Work out the finished part from the listing and answer in its coordinate system (mm). Round coordinates to 2 decimals unless told otherwise and drop trailing zeros. Write each loop counter-clockwise with the first axis right and the second up, starting at its lowest first coordinate (ties: lowest second). Pieces come first, ordered by that corner, then holes. Notation, with made-up numbers: (44, -13.5) -> (72, -13.5) arc R12 ccw to (72, 2.5) -> close; hole circle Ø4 at (-21, 50.5). An arc over 180 degrees is marked (long way). One line per item, written item: value.
Autodesk Inventor part; units mm, degrees
ref_plane "YZ Plane" through (0, 0, 0) normal (1, 0, 0) x (0, 1, 0)
ref_plane "XZ Plane" through (0, 0, 0) normal (0, 1, 0) x (-1, 0, 0)
ref_plane "XY Plane" through (0, 0, 0) normal (0, 0, 1) x (1, 0, 0)
sketch "Sketch_16" plane through (0, 0, 0) normal (0, 0, 1) x (1, 0, 0)
  line L0 (391, 0) -> (7, 0)
  line L1 (7, 0) -> (7, 6)
  line L2 (7, 6) -> (391, 6)
  line L3 (391, 6) -> (391, 0)
  line L4 (391, 0) -> (7, 0)
revolve "Revolution1" add sketch "Sketch_16" angle 360 about axis through (391, 0, 0) along (1, 0, 0)
thread "Thread1"
sketch "Sketch_23" plane through (0, 0, 0) normal (0, 0, 1) x (1, 0, 0)
  line L0 (7, 0) -> (0, 0)
  line L1 (0, 0) -> (0, 3.5)
  line L2 (0, 3.5) -> (0.5, 4)
  line L3 (0.5, 4) -> (6.7, 4)
  arc A0 (6.7, 4) -> (7, 4.3) centre (6.7, 4.3) ccw
  line L4 (7, 4.3) -> (7, 0)
  line L5 (7, 0) -> (0, 0)
revolve "Revolution2" add sketch "Sketch_23" angle 360 about axis through (7, 0, 0) along (1, 0, 0)
sketch "Sketch_4" plane through (0, 0, 0) normal (0, 0, 1) x (1, 0, 0)
  line L0 (420, 0) -> (391, 0)
  line L1 (391, 0) -> (391, 4.3)
  arc A0 (391, 4.3) -> (391.3, 4) centre (391.3, 4.3) ccw
  line L2 (391.3, 4) -> (400, 4)
  line L3 (400, 4) -> (400, 2.8)
  arc A1 (400, 2.8) -> (400.3, 2.5) centre (400.3, 2.8) ccw
  line L4 (400.3, 2.5) -> (419.5, 2.5)
  line L5 (419.5, 2.5) -> (420, 2)
  line L6 (420, 2) -> (420, 0)
  line L7 (420, 0) -> (391, 0)
revolve "Revolution3" add sketch "Sketch_4" angle 360 about axis through (420, 0, 0) along (1, 0, 0)
sketch "Sketch_8" plane through (420, 0, 0) normal (1, 0, 0) x (0, 0, -1)
  line L0 (-2.5, -6) -> (-1.5, -6)
  line L1 (-1.5, -6) -> (-1.5, 6)
  line L2 (-1.5, 6) -> (-2.5, 6)
  line L3 (-2.5, 6) -> (-2.5, -6)
extrude "Extrusion1" cut sketch "Sketch_8" against normal blind 7
properties part number "MTSBRK12-420-F7-R8-T9-Q8-S20-E5-FE0-FW7-FY1" material "Steel, Carbon"
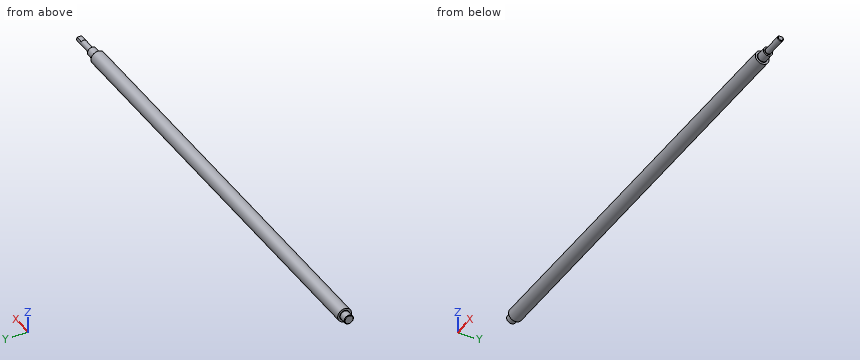
(1) Flat-ended cylindrical pins translate along their axes: pin 1 Ø2 at (y, z) = (-3, -4.5) entering from +X; pin 2 Ø6 at (x, z) = (208, 3.5) entering from +Y; pin 3 Ø1.5 at (y, z) = (-4, 2.5) entering from +X. Find the tip coordinate at first contact, or state that the pin passes through.
Reported:
pin 1: stops at x = 391
pin 2: stops at y = 5.98
pin 3: stops at x = 400
(2) Consider probe 1 along X at (y, z) = (4.75, -3); probe 2 along Y at (x, z) = (268, -4.5); probe 3 along Y at (x, z) = (77.5, -1). Determine where each line is inside the solid, lowest interval first.
Reported:
probe 1: x = 7 to 391
probe 2: y = -3.97 to 3.97
probe 3: y = -5.92 to 5.92
(3) Find section A-A on x = 287. Give the vertices of the cut face in (y, z), plus the area to 3 significant figures.
Reported:
outline: circle Ø12 at (0, 0)
area: 113 mm2
